from build123d import *

# Parameters (mm, degrees)
BOSS_EXTRUDE1_DEPTH = 7
CUT_EXTRUDE1_DEPTH  = 6
CUT_EXTRUDE2_DEPTH  = 8
BOSS_EXTRUDE2_DEPTH = 10
SKETCH5_W           = 2.4
SKETCH5_H           = 0.9
BOSS_EXTRUDE3_DEPTH = 0.8
SKETCH6_W           = 2.4
SKETCH6_H           = 0.9
BOSS_EXTRUDE4_DEPTH = 0.8
SKETCH7_R           = 0.5
CUT_EXTRUDE3_DEPTH  = 1


with BuildPart() as part:
    # Sketch1 → Boss-Extrude1 (new body)
    with BuildSketch(Plane(origin=(0, 0, 0), x_dir=(1, 0, 0), z_dir=(0, 1, 0))):
        Polygon((-20.25, 14.738772175), (-15.362506196, 19.75), (15.362506196, 19.75), (20.25, 14.738772175), (20.25, -14.738772175), (15.362506196, -19.75), (-15.362506196, -19.75), (-20.25, -14.738772175), align=None)
    extrude(amount=BOSS_EXTRUDE1_DEPTH)

    # Sketch2 → Cut-Extrude1 (cut)
    with BuildSketch(Plane.XZ):
        Polygon((14.940951585, 18.75), (-14.940951585, 18.75), (-19.25, 14.331861751), (-19.25, -14.331861751), (-14.940951585, -18.75), (14.940951585, -18.75), (19.25, -14.331861751), (19.25, 14.331861751), align=None)
    extrude(amount=-CUT_EXTRUDE1_DEPTH, mode=Mode.SUBTRACT)

    # Sketch3 → Cut-Extrude2 (cut, through all)
    with BuildSketch(Plane(origin=(0, 7, 0), x_dir=(1, 0, 0), z_dir=(0, 1, 0))):
        Polygon((14.262506196, 19.75), (1.762506196, 19.75), (1.762506196, 16.137014737), (0.777606409, 16.137014737), (0.777606409, 12.137014737), (1.762506196, 12.137014737), (1.762506196, 10.75), (14.262506196, 10.75), align=None)
    extrude(amount=-CUT_EXTRUDE2_DEPTH, mode=Mode.SUBTRACT)

    # Sketch4 → Boss-Extrude2 (add)
    with BuildSketch(Plane.XZ.offset(-6)):
        Polygon((0.762506196, -18.75), (1.762506196, -18.75), (1.762506196, -16.137014737), (0.777606409, -16.137014737), (0.777606409, -12.137014737), (1.762506196, -12.137014737), (1.762506196, -10.75), (14.262506196, -10.75), (14.262506196, -18.75), (15.262506196, -18.75), (15.262506196, -9.75), (0.762506196, -9.75), (0.762506196, -11.137014737), (-0.222393591, -11.137014737), (-0.222393591, -17.137014737), (0.762506196, -17.137014737), align=None)
    extrude(amount=BOSS_EXTRUDE2_DEPTH)

    # Sketch5 → Boss-Extrude3 (add)
    with BuildSketch(Plane.ZY.offset(20.25)):
        with Locations((-11.369651621, 3.25)):
            Rectangle(SKETCH5_W, SKETCH5_H)
        with Locations((11.369651621, 3.25)):
            Rectangle(SKETCH5_W, SKETCH5_H)
    extrude(amount=BOSS_EXTRUDE3_DEPTH)

    # Sketch6 → Boss-Extrude4 (add)
    with BuildSketch(Plane(origin=(20.25, 0, 0), x_dir=(0, 0, -1), z_dir=(1, 0, 0))):
        with Locations((-11.369651621, 3.25)):
            Rectangle(SKETCH6_W, SKETCH6_H)
        with Locations((11.369651621, 3.25)):
            Rectangle(SKETCH6_W, SKETCH6_H)
    extrude(amount=BOSS_EXTRUDE4_DEPTH)

    # Sketch7 → Cut-Extrude3 (cut)
    with BuildSketch(Plane(origin=(0, 7, 0), x_dir=(1, 0, 0), z_dir=(0, 1, 0))):
        with Locations((-4.884098743, -10.5)):
            Circle(SKETCH7_R)
        with Locations((-7.884098743, -10.5)):
            Circle(SKETCH7_R)
        with Locations((-10.884098743, -10.5)):
            Circle(SKETCH7_R)
        with Locations((-13.884098743, -10.5)):
            Circle(SKETCH7_R)
        with Locations((-7.884098743, -7.5)):
            Circle(SKETCH7_R)
        with Locations((-10.884098743, -7.5)):
            Circle(SKETCH7_R)
        with Locations((-13.884098743, -7.5)):
            Circle(SKETCH7_R)
        with Locations((-7.884098743, -4.5)):
            Circle(SKETCH7_R)
        with Locations((-10.884098743, -4.5)):
            Circle(SKETCH7_R)
        with Locations((-13.884098743, -4.5)):
            Circle(SKETCH7_R)
        with Locations((-7.884098743, -1.5)):
            Circle(SKETCH7_R)
        with Locations((-10.884098743, -1.5)):
            Circle(SKETCH7_R)
        with Locations((-13.884098743, -1.5)):
            Circle(SKETCH7_R)
        with Locations((-7.884098743, 1.5)):
            Circle(SKETCH7_R)
        with Locations((-10.884098743, 1.5)):
            Circle(SKETCH7_R)
        with Locations((-13.884098743, 1.5)):
            Circle(SKETCH7_R)
        with Locations((-7.884098743, 4.5)):
            Circle(SKETCH7_R)
        with Locations((-10.884098743, 4.5)):
            Circle(SKETCH7_R)
        with Locations((-13.884098743, 4.5)):
            Circle(SKETCH7_R)
        with Locations((-7.884098743, 7.5)):
            Circle(SKETCH7_R)
        with Locations((-10.884098743, 7.5)):
            Circle(SKETCH7_R)
        with Locations((-13.884098743, 7.5)):
            Circle(SKETCH7_R)
        with Locations((-7.884098743, 10.5)):
            Circle(SKETCH7_R)
        with Locations((-10.884098743, 10.5)):
            Circle(SKETCH7_R)
        with Locations((-13.884098743, 10.5)):
            Circle(SKETCH7_R)
        with Locations((-4.884098743, -7.5)):
            Circle(SKETCH7_R)
        with Locations((-4.884098743, -4.5)):
            Circle(SKETCH7_R)
        with Locations((-4.884098743, -1.5)):
            Circle(SKETCH7_R)
        with Locations((-4.884098743, 1.5)):
            Circle(SKETCH7_R)
        with Locations((-4.884098743, 4.5)):
            Circle(SKETCH7_R)
        with Locations((-4.884098743, 7.5)):
            Circle(SKETCH7_R)
        with Locations((-4.884098743, 10.5)):
            Circle(SKETCH7_R)
    extrude(amount=-CUT_EXTRUDE3_DEPTH, mode=Mode.SUBTRACT)


solid = part.part
Geometry check sheet. Reference: the model listing, model coordinates, mm. A direction names the side the tool comes from. Give positions to 0.01 mm unless a question says otherwise; leave off trailing zeros. Loops run counter-clockwise (first coordinate to the right, second up) from the corner with the lowest first, then second, coordinate; pieces in that order, holes last. Notation, with made-up numbers: (6.25, 1) -> (38.25, 1) arc R32 ccw to (38.25, 36) -> close; hole circle Ø2 at (20, 83). An arc over 180 degrees is marked (long way). Answer in a Markdown table with one row per item. Add a question column.
1) Cross-section at A-A on y = -1.25. Record the boundary of the cut face in (x, z), and give its area (3 significant figures).
2) Cross-section at C-C on x = 2.5. Record the boundary of the cut face in (y, z), and give its area (3 significant figures).
3) Gauge pin test, flat ends, axial feed: P1, Ø1, axis at y = 5.5, z = -8, coming from the +X side; P2, Ø0.9, axis at x = -20.5, y = 3.5, coming from the +Z side; P3, Ø0.9, axis at x = -21, z = -11.5, coming from the -Y side. Record the tip position at first contact, or that the pin passes through.
4) Cross-section at D-D on x = -6. Record the boundary of the cut face in (y, z).
5) Material ranges on probe 1 along X at (y, z) = (3.25, -13.5); probe 2 along X at (y, z) = (6.4, 7.5); probe 3 along X at (y, z) = (5.25, 2), recorded low to high. Write a range as from..to.
6) Cross-section at B-B on z = -1.5. Record the boundary of the cut face in (x, y), and give its area (3 significant figures).
7) Set-up check for faces 4 (the face through (15, -2, -18.75)), 5 (the face through (15, 3, -19.75)), 6 (the face through (0.763, 1, -18)), 7 (the face through (1.763, 2, -11)): record each of +Z, -Z, +X, -X, +Y, -Y from which the full face is reachable in a straight line by a thin tool's end or side.
8) Draft check along X on faces 1 (the face through (-21.05, 3, -11)), 2 (the face through (8, 2, -10.75)), 3 (the face through (1, -2, -18.75)). Enter one of: pulls with the +X half, pulls with the -X half, needs draft (parallel to the pull), parting line crosses it, or undercut.
Outcome:
| question | item | result |
|---|---|---|
| 1 | outline | (-0.22, -17.14) -> (0.76, -17.14) -> (0.76, -18.75) -> (1.76, -18.75) -> (1.76, -16.14) -> (0.78, -16.14) -> (0.78, -12.14) -> (1.76, -12.14) -> (1.76, -10.75) -> (14.26, -10.75) -> (14.26, -18.75) -> (15.26, -18.75) -> (15.26, -9.75) -> (0.76, -9.75) -> (0.76, -11.14) -> (-0.22, -11.14) -> close |
| 1 | area | 32.5 mm^2 |
| 2 | outline | (-4, -10.75) -> (7, -10.75) -> (7, 19.75) -> (0, 19.75) -> (0, 18.75) -> (6, 18.75) -> (6, -9.75) -> (-4, -9.75) -> close |
| 2 | area | 46.5 mm^2 |
| 3 | P1 | stops at x = 20.25 |
| 3 | P2 | stops at z = 14.94 |
| 3 | P3 | stops at y = 2.8 |
| 4 | outline | (0, -19.75) -> (7, -19.75) -> (7, 19.75) -> (0, 19.75) -> (0, 18.75) -> (6, 18.75) -> (6, -18.75) -> (0, -18.75) -> close |
| 5 | probe 1 | x = -20.25..-19.25, -0.22..0.78, 14.26..15.26, 19.25..20.25 |
| 5 | probe 2 | x = -20.25..-14.38, -13.38..-11.38, -10.38..-8.38, -7.38..-5.38, -4.38..20.25 |
| 5 | probe 3 | x = -20.25..-19.25, 19.25..20.25 |
| 6 | outline | (-20.25, 0) -> (-19.25, 0) -> (-19.25, 6) -> (-14.38, 6) -> (-14.38, 7) -> (-20.25, 7) -> close; (-13.38, 6) -> (-11.38, 6) -> (-11.38, 7) -> (-13.38, 7) -> close; (-10.38, 6) -> (-8.38, 6) -> (-8.38, 7) -> (-10.38, 7) -> close; (-7.38, 6) -> (-5.38, 6) -> (-5.38, 7) -> (-7.38, 7) -> close; (-4.38, 6) -> (19.25, 6) -> (19.25, 0) -> (20.25, 0) -> (20.25, 7) -> (-4.38, 7) -> close |
| 6 | area | 48.5 mm^2 |
| 7 | face 4 | -Z, +X, -X, -Y |
| 7 | face 5 | -Z, +X, -X, +Y, -Y |
| 7 | face 6 | -Y |
| 7 | face 7 | -Z, +Y, -Y |
| 8 | face 1 | pulls with the -X half |
| 8 | face 2 | undercut |
| 8 | face 3 | needs draft |
